```python
from build123d import *

# Parameters (mm, degrees)
F0_R     = 14.2875
F1_DEPTH = 41.148
F0_R_2   = 7.298311
F2_DEPTH = 11.176
F3_R     = 5.08
F4_R     = 3.048
F6_DEPTH = 2.794


with BuildPart() as f1:
    # F0 (on Front) → F1 (new body)
    with BuildSketch(Plane.XZ):
        with BuildLine():
            ThreePointArc((-13.16432, -21.722355), (12.465678, -22.130677), (25.4, 0))
            ThreePointArc((25.4, 0), (12.465678, 22.130677), (-13.16432, 21.722355))
            ThreePointArc((-13.16432, 21.722355), (-25.4, 0), (-13.16432, -21.722355))
        make_face()
        Circle(F0_R, mode=Mode.SUBTRACT)
    extrude(amount=F1_DEPTH)

    # F0 (on Front) → F2 (join)
    with BuildSketch(Plane.XZ):
        with BuildLine():
            ThreePointArc((-13.16432, 21.722355), (12.465678, 22.130677), (25.4, 0))
            ThreePointArc((25.4, 0), (12.465678, -22.130677), (-13.16432, -21.722355))
            Line((-13.16432, -21.722355), (32.706421, -51.803458))
            ThreePointArc((32.706421, -51.803458), (51.531426, -52.981963), (62.14277, -37.388084))
            Line((62.14277, -37.388084), (62.14277, 37.388084))
            ThreePointArc((62.14277, 37.388084), (51.531426, 52.981963), (32.706421, 51.803458))
            Line((32.706421, 51.803458), (-13.16432, 21.722355))
        make_face()
        with Locations((43.15309, -35.873311)):
            Circle(F0_R_2, mode=Mode.SUBTRACT)
        with Locations((43.15309, 35.873311)):
            Circle(F0_R_2, mode=Mode.SUBTRACT)
    extrude(amount=F2_DEPTH)

    # F3
    f3_edges = [f1.edges().sort_by_distance(p)[0] for p in [
        (-14.2875, -41.148, 0),
    ]]
    fillet(f3_edges, radius=F3_R)

    # F4
    f4_edges = [f1.edges().sort_by_distance(p)[0] for p in [
        (-25.4, -41.148, 0),
    ]]
    fillet(f4_edges, radius=F4_R)

    # F5 (on Top) → F6 (join, symmetric)
    with BuildSketch(Plane.XY):
        Polygon((59.404932, -11.267408), (25.343085, -11.20039), (25.343085, -36.381185), align=None)
    extrude(amount=F6_DEPTH, both=True)


solid = f1.part
```
Check sheet for the modelled part. Datum: model origin and axes. Units: mm. Round coordinates to 2 decimals unless told otherwise and drop trailing zeros. Order: outer loops, then holes, each group sorted by start corner. A loop starts at its lowest first (then second) coordinate and runs counter-clockwise, first axis right, second up. Notation, with made-up numbers: (34, 14) -> (56, 14) arc R27 ccw to (56, 41) -> close; hole circle Ø11 at (-36, -28). An arc over 180 degrees is marked (long way). One line per item, written item: value. Start each with the question number.
Q1. Gauge pin test, flat ends, axial feed: pin 1 Ø12 at (y, z) = (-35, -2) entering from +X; pin 2 Ø5 at (y, z) = (-7, -40) entering from +X; pin 3 Ø0.9 at (y, z) = (-22.5, 2) entering from -X. Record the tip position at first contact, or that the pin passes through.
Q2. Cross-section at A-A (z = -30). Record the boundary of the cut face in (x, y), and give its area (3 significant figures).
Q3. Mould release check, pull along Z, two halves, no side actions. Record for faces 1 (the face through (-14.274, -17.782, 0.628)), 2 (the face through (35.86, -5.51, 36.19)), 3 (the face through (38, -21, 2.794)), 4 (the face through (38, -21, -2.794)): pulls with the +Z half, pulls with the -Z half, needs draft (parallel to the pull), parting line crosses it, or undercut.
Q4. Thickness scan on line 1 (Z direction, x = 0, y = -15.5); line 2 (Z direction, x = 45, y = -7.5); line 3 (X direction, y = -2, z = -4). Record the ranges inside material, lowest first.
Q5. Cross-section at B-B (x = 43.5). Record the boundary of the cut face in (y, z), and give its area (3 significant figures).
Completed:
1. pin 1: stops at x = 35.35
1. pin 2: stops at x = 62.13
1. pin 3: stops at x = -25.35
2. outline: (-0.54, -11.18) -> (38.82, -11.18) -> (38.82, 0) -> (-0.54, 0) -> close; (47.49, -11.18) -> (62.14, -11.18) -> (62.14, 0) -> (47.49, 0) -> close
2. area: 604 mm²
3. face 1: undercut
3. face 2: undercut
3. face 3: pulls with the +Z half
3. face 4: pulls with the -Z half
4. line 1: z = -25.4 to -14.29, 14.29 to 25.4
4. line 2: z = -54.83 to -42.93, -28.81 to 28.81, 42.93 to 54.83
4. line 3: x = -25.08 to -13.72, 13.72 to 62.14
5. outline: (-22.99, -2.79) -> (-11.24, -2.79) -> (-11.24, 2.79) -> (-22.99, 2.79) -> close; (-11.18, -54.92) -> (0, -54.92) -> (0, -43.16) -> (-11.18, -43.16) -> close; (-11.18, -28.58) -> (0, -28.58) -> (0, 28.58) -> (-11.18, 28.58) -> close; (-11.18, 43.16) -> (0, 43.16) -> (0, 54.92) -> (-11.18, 54.92) -> close
5. area: 967 mm²
